For this review, take the finished solid that the model builds, in its own axes (mm). Coordinates: 2 decimals unless noted, no trailing zeros. Order: outer loops, then holes, each group sorted by start corner. A loop starts at its lowest first (then second) coordinate and runs counter-clockwise, first axis right, second up. Notation, with made-up numbers: (36, 22.25) -> (60, 22.25) arc R12 cw to (60, 28.25) -> close; hole circle Ø3 at (61.25, 47). An arc over 180 degrees is marked (long way). Return JSON: item names as keys, results as strings. Group by question number.
Item 1: Take a section at B-B (x = 0). Write out the cut boundary in (y, z).
Item 2: Take a section at C-C (y = 2.7). Write out the cut boundary in (x, z).
Item 3: For line 1 along Z through (x, y) = (0, 3.1); line 2 along Z through (x, y) = (-0.75, 1.9); line 3 along Z through (x, y) = (-1.5, 1.95), list the stretches that pass through material, from the lowest coordinate up.
Item 4: Draft analysis for pull direction Z (two halves, no side actions). For faces 1 (the flat face through (0, 0, 5)), 2 (the cylindrical face through (-2.38, 2.35, 10.74)), 3 (the cylindrical face through (-0.56, 2.41, 8.89)), 4 (the cylindrical face through (-2.285, 2.415, 3.584)), state which applies: +Z half, -Z half, draft (parallel to the pull), parting line (faces both ways), or undercut.
Item 5: Take a section at D-D (x = -8). Write out the cut boundary in (y, z).
Item 6: Take a section at A-A (z = 0). Write out the cut boundary in (x, y).
Item 7: Insertion check: pin 1 (2 mm diameter, centred on x = 3, y = 3.5, fed in from +Z); pin 2 (2 mm diameter, centred on x = 1.5, y = 1.5, fed in from -Z); pin 3 (1 mm diameter, centred on y = 3.5, z = 7, fed in from +X). Each pin has a flat end and moves straight along its axis. Give the tip position at first contact, or say it passes through.
```python
from build123d import *

# Parameters (mm, degrees)
SKETCH1_R           = 11
BOSS_EXTRUDE1_DEPTH = 4.7625
SKETCH2_R           = 1.05
CUT_EXTRUDE1_DEPTH  = 5.7625
SKETCH3_R           = 4.25
CUT_EXTRUDE2_DEPTH  = 5.7625


with BuildPart() as part:
    # Sketch1 → Boss-Extrude1 (new body)
    with BuildSketch(Plane(origin=(0, 0, 0), x_dir=(1, 0, 0), z_dir=(0, 1, 0))):
        Circle(SKETCH1_R)
    extrude(amount=BOSS_EXTRUDE1_DEPTH)

    # Sketch2 → Cut-Extrude1 (cut, through all)
    with BuildSketch(Plane(origin=(0, 4.7625, 0), x_dir=(-1, 0, 0), z_dir=(0, 1, 0))):
        with Locations((0, 8)):
            Circle(SKETCH2_R)
        with Locations((8, 0)):
            Circle(SKETCH2_R)
        with Locations((0, -8)):
            Circle(SKETCH2_R)
        with Locations((-8, 0)):
            Circle(SKETCH2_R)
    extrude(amount=-CUT_EXTRUDE1_DEPTH, mode=Mode.SUBTRACT)

    # Sketch3 → Cut-Extrude2 (cut, through all)
    with BuildSketch(Plane(origin=(0, 4.7625, 0), x_dir=(-1, 0, 0), z_dir=(0, 1, 0))):
        Circle(SKETCH3_R)
    extrude(amount=-CUT_EXTRUDE2_DEPTH, mode=Mode.SUBTRACT)


solid = part.part
```
Findings below:
{
 "1": {"outline": "(0, -11) -> (4.76, -11) -> (4.76, -9.05) -> (0, -9.05) -> close; (0, -6.95) -> (4.76, -6.95) -> (4.76, -4.25) -> (0, -4.25) -> close; (0, 4.25) -> (4.76, 4.25) -> (4.76, 6.95) -> (0, 6.95) -> close; (0, 9.05) -> (4.76, 9.05) -> (4.76, 11) -> (0, 11) -> close"},
 "2": {"outline": "circle Ø22 at (0, 0); hole circle Ø2.1 at (-8, 0); hole circle Ø8.5 at (0, 0); hole circle Ø2.1 at (0, -8); hole circle Ø2.1 at (0, 8); hole circle Ø2.1 at (8, 0)"},
 "3": {"line 1": "z = -11 to -9.05, -6.95 to -4.25, 4.25 to 6.95, 9.05 to 11", "line 2": "z = -10.97 to -8.73, -7.27 to -4.18, 4.18 to 7.27, 8.73 to 10.97", "line 3": "z = -10.9 to -3.98, 3.98 to 10.9"},
 "4": {"face 1": "draft", "face 2": "parting line", "face 3": "undercut", "face 4": "undercut"},
 "5": {"outline": "(0, -7.55) -> (4.76, -7.55) -> (4.76, -1.05) -> (0, -1.05) -> close; (0, 1.05) -> (4.76, 1.05) -> (4.76, 7.55) -> (0, 7.55) -> close"},
 "6": {"outline": "(-11, 0) -> (-9.05, 0) -> (-9.05, 4.76) -> (-11, 4.76) -> close; (-6.95, 0) -> (-4.25, 0) -> (-4.25, 4.76) -> (-6.95, 4.76) -> close; (4.25, 0) -> (6.95, 0) -> (6.95, 4.76) -> (4.25, 4.76) -> close; (9.05, 0) -> (11, 0) -> (11, 4.76) -> (9.05, 4.76) -> close"},
 "7": {"pin 1": "stops at z = 10.82", "pin 2": "stops at z = -10.99", "pin 3": "stops at x = 8.87"}
}
